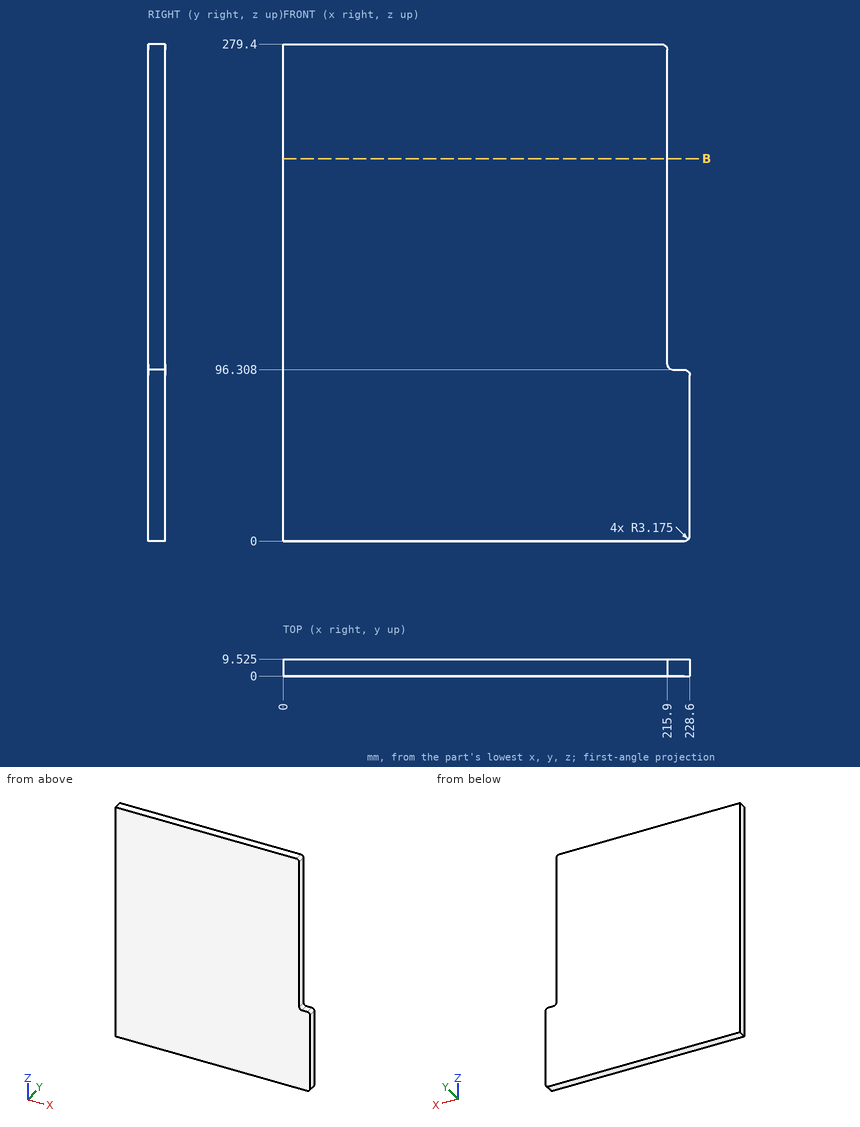
The drawing under review shows one solid part. Ordinate dimensions are in mm from its lowest x, y, z. Coordinates: 2 decimals unless noted, no trailing zeros. Loops run counter-clockwise (first coordinate to the right, second up) from the corner with the lowest first, then second, coordinate; pieces in that order, holes last.
Item 1: Wall thickness on L1, parallel to X at y = 1, z = 181.5; L2, parallel to X at y = 6.5, z = 98; L3, parallel to Z at x = 218, y = 5.5 (1 decimal): over which ranges is each line inside the solid? List them lowest first.
Completed:
L1: x = 0 to 215.9
L2: x = 0 to 216.27
L3: z = 0 to 96.5
Item 2: Add section B-B (z = 215). Write out the cut boundary in (x, y) (1 decimal).
Completed:
outline: (0, 0) - (215.9, 0) - (215.9, 9.5) - (0, 9.5) - close
Item 3: Clearance check with a flat-ended pin moving along its axis: pin 1 (5 mm diameter, centred on y = 5, z = 154, fed in from +X). State where the tip first meets the part, or that it passes through.
Completed:
pin 1: stops at x = 215.9
